Could you check a few things on this model? Use its own coordinates, in mm. Face numbers are marked on the shaded views. A direction names the side the tool comes from. Round coordinates to 2 decimals unless told otherwise and drop trailing zeros. Loops run counter-clockwise (first coordinate to the right, second up) from the corner with the lowest first, then second, coordinate; pieces in that order, holes last. Notation, with made-up numbers: (-15, 37.5) -> (43, 37.5) arc R16 cw to (43, 43.5) -> close; hole circle Ø7 at (59.5, -9). An arc over 180 degrees is marked (long way). One line per item, written item: value.
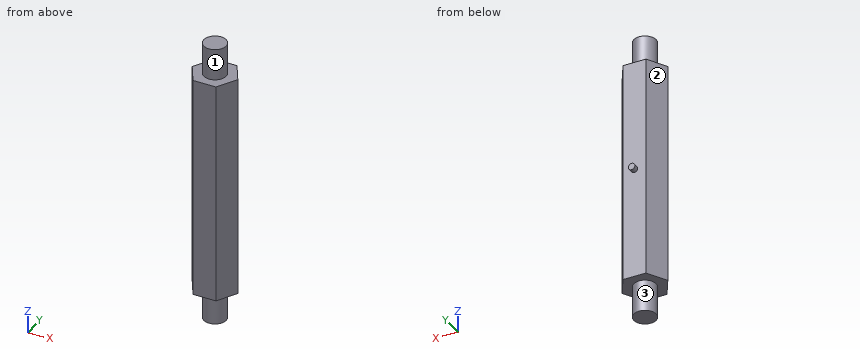
```python
from build123d import *

# Parameters (mm, degrees)
BOSS_EXTRUDE1_DEPTH = 53.975
SKETCH2_R           = 5.3975
BOSS_EXTRUDE2_DEPTH = 15.24
SKETCH3_R           = 1.5875
BOSS_EXTRUDE3_DEPTH = 2.54


with BuildPart() as part:
    # Sketch1 → Boss-Extrude1 (new body)
    with BuildSketch(Plane.XY):
        Polygon((5.499261314, 9.525), (-5.499261314, 9.525), (-10.998522628, 0), (-5.499261314, -9.525), (5.499261314, -9.525), (10.998522628, 0), align=None)
    extrude(amount=BOSS_EXTRUDE1_DEPTH)

    # Sketch2 → Boss-Extrude2 (add)
    with BuildSketch(Plane.XY.offset(53.975)):
        with Locations(Location((0, 0, 0), (0, 0, 180))):
            Circle(SKETCH2_R)
    extrude(amount=BOSS_EXTRUDE2_DEPTH)

    # Mirror1: part across plane


with BuildPart() as part_1:
    add(part.part)
    add(part.part.mirror(Plane.XY))

    # Sketch3 → Boss-Extrude3 (add)
    with BuildSketch(Plane(origin=(0, 9.525, 0), x_dir=(1, 0, 0), z_dir=(0, 1, 0))):
        with Locations(Location((0, 0, 0), (0, 0, 90))):
            Circle(SKETCH3_R)
    extrude(amount=BOSS_EXTRUDE3_DEPTH)


solid = part_1.part
```
Item 1: If we section it at D-D on z = 52: List the corners of the cut face in (x, y) for me (3 decimals).
Output:
outline: (-10.999, 0) -> (-5.499, -9.525) -> (5.499, -9.525) -> (10.999, 0) -> (5.499, 9.525) -> (-5.499, 9.525) -> close
Item 2: Will these pins go through, and if not, where does the flat tip stop? pin 1 Ø4 at (y, z) = (-5.5, -29) entering from +X; pin 2 Ø4 at (y, z) = (8.5, 43) entering from +X; pin 3 Ø1 at (x, y) = (5, 3.5) entering from +Z (3 decimals).
Output:
pin 1: stops at x = 8.98
pin 2: stops at x = 7.25
pin 3: stops at z = 53.975
Item 3: If we section it at B-B on x = 0: List the corners of the cut face in (y, z) for me (1 decimal).
Output:
outline: (-9.5, -54) -> (-5.4, -54) -> (-5.4, -69.2) -> (5.4, -69.2) -> (5.4, -54) -> (9.5, -54) -> (9.5, -1.6) -> (12.1, -1.6) -> (12.1, 1.6) -> (9.5, 1.6) -> (9.5, 54) -> (5.4, 54) -> (5.4, 69.2) -> (-5.4, 69.2) -> (-5.4, 54) -> (-9.5, 54) -> close
Item 4: I need wall thicknesses on line 1 (Y direction, x = -5, z = -42.5) (3 decimals); line 2 (Z direction, x = -7.25, y = -0.5) (3 decimals); line 3 (Y direction, x = -0.25, z = 61). Which ranges of each line are inside material? Lowest first, please. Write a range as from..to.
Output:
line 1: y = -9.525..9.525
line 2: z = -53.975..53.975
line 3: y = -5.39..5.39
Item 5: For the marked faces 1, 2 and 3, which set-ups out of +Z, -Z, +X, -X, +Y, -Y let a thin tool reach every point of the face, with its end or its side?
Output:
face 1: +Z
face 2: +Z, -Z, -X, +Y
face 3: -Z
Item 6: If we section it at C-C on y = 2.25: List the corners of the cut face in (x, z) for me (3 decimals).
Output:
outline: (-9.699, -53.975) -> (-4.906, -53.975) -> (-4.906, -69.215) -> (4.906, -69.215) -> (4.906, -53.975) -> (9.699, -53.975) -> (9.699, 53.975) -> (4.906, 53.975) -> (4.906, 69.215) -> (-4.906, 69.215) -> (-4.906, 53.975) -> (-9.699, 53.975) -> close
Item 7: If we section it at A-A on z = 0: List the corners of the cut face in (x, y) for me (1 decimal).
Output:
outline: (-11, 0) -> (-5.5, -9.5) -> (5.5, -9.5) -> (11, 0) -> (5.5, 9.5) -> (1.6, 9.5) -> (1.6, 12.1) -> (-1.6, 12.1) -> (-1.6, 9.5) -> (-5.5, 9.5) -> close
